```python
from build123d import *

# Parameters (mm, degrees)
CYLINDER018_R     = 50
CYLINDER018_DEPTH = 10
CYLINDER017_R     = 8
CYLINDER017_DEPTH = 5


with BuildPart() as cylinder019:
    # Cylinder018 → Cylinder018 (new body)
    with BuildSketch(Plane.XY):
        Circle(CYLINDER018_R)
    extrude(amount=CYLINDER018_DEPTH)


with BuildPart() as common:
    # Cylinder017 → Cylinder017 (new body)
    with BuildSketch(Plane(origin=(0, 51, 0), x_dir=(1, 0, 0), z_dir=(0, 0, 1))):
        Circle(CYLINDER017_R)
    extrude(amount=CYLINDER017_DEPTH)

    # Common: intersect Cylinder019
    add(cylinder019.part, mode=Mode.INTERSECT)


solid = common.part
```
Verification items for the finished model (mm, model axes). Give positions to 0.01 mm unless a question says otherwise; leave off trailing zeros. Loops run counter-clockwise (first coordinate to the right, second up) from the corner with the lowest first, then second, coordinate; pieces in that order, holes last. Notation, with made-up numbers: M -27,69 L 28,69 A11 cw 28,78 Z; hole C 54.25,-37.5 d7. An arc over 180 degrees is marked long. Return JSON: item names as keys, results as strings.
1) Section check C-C, the plane x = -4.5. Enter the section's corners in (y, z), and give its area (3 significant figures).
Findings:
{"outline": "M 44.39,0 L 49.8,0 L 49.8,5 L 44.39,5 Z", "area": "27.1 mm2"}
2) Section check A-A, the plane z = 3.1. Enter the section's corners in (x, y), and give its area (3 significant figures).
Findings:
{"outline": "M -7.83,49.38 A8 ccw 7.83,49.38 A50 ccw Z", "area": "81.3 mm2"}
3) Material ranges on L1, parallel to X at y = 48.5, z = 1.05; L2, parallel to X at y = 49, z = 3.95; L3, parallel to Y at x = 5.25, z = 1.1, recorded low to high. Write a range as [from, to].
Findings:
{"L1": "x = [-7.6, 7.6]", "L2": "x = [-7.75, 7.75]", "L3": "y = [44.96, 49.72]"}
4) Gauge pin test, flat end, axial feed: P1, Ø3, axis at y = 45.5, z = 3.5, coming from the -X side. Record the tip position at first contact, or that the pin passes through.
Findings:
{"P1": "stops at x = -6.93"}
5) Section check B-B, the plane y = 45. Enter the section's corners in (x, z), and give its area (3 significant figures).
Findings:
{"outline": "M -5.29,0 L 5.29,0 L 5.29,5 L -5.29,5 Z", "area": "52.9 mm2"}
